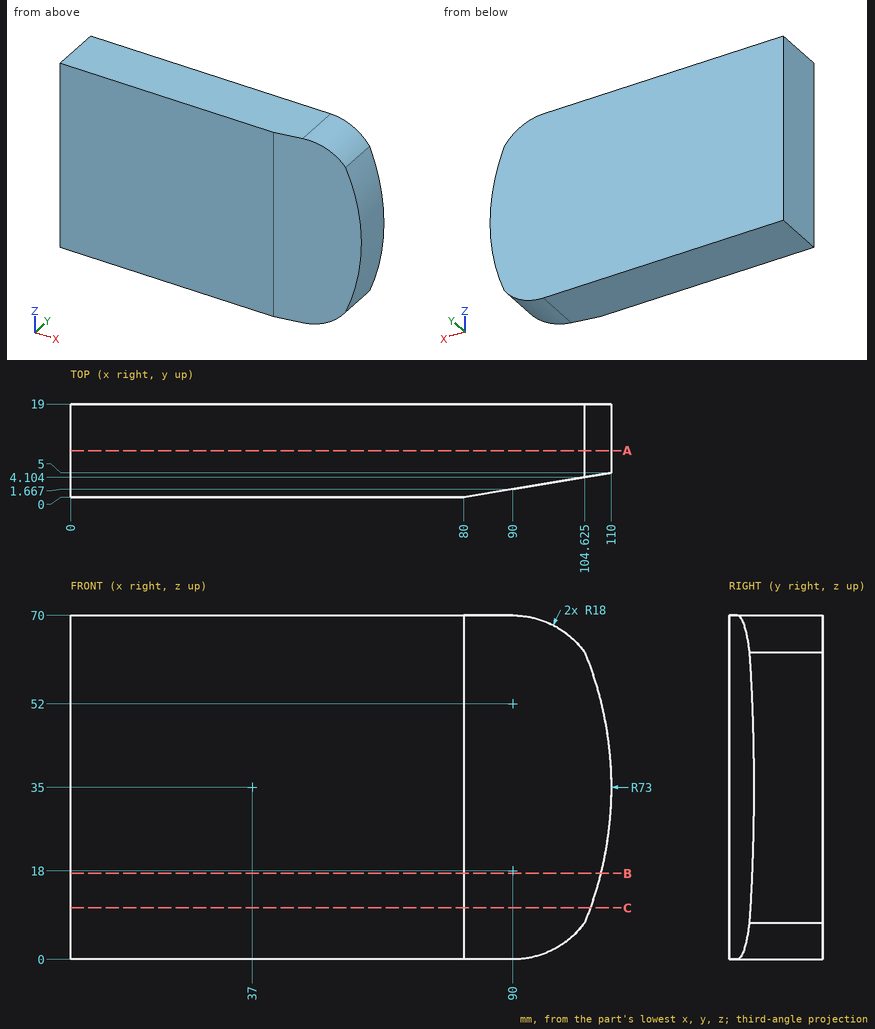
Design review of the part shown in the three views and the two pictorial views. Dimensions are in mm from the part's minimum x, y and z. Give positions to 0.01 mm unless a question says otherwise; leave off trailing zeros. Loops run counter-clockwise (first coordinate to the right, second up) from the corner with the lowest first, then second, coordinate; pieces in that order, holes last. Notation, with made-up numbers: (82.5, 37.25) -> (112.5, 37.25) arc R34 cw to (112.5, 70.25) -> close; hole circle Ø7 at (-6.5, 24.25). An arc over 180 degrees is marked (long way). Put each result on its own line as item: value. Start each with the question number.
1. We need section C-C on z = 10.5. State the section outline as (x, y) points (1 decimal), then the cut area to 3 significant figures.
2. We need section A-A on y = 9.5. State the section outline as (x, z) points (1 decimal), then the cut area to 3 significant figures.
3. Wall thickness on probe 1 along Y at (x, z) = (81.5, 38.5); probe 2 along X at (y, z) = (5, 56.5); probe 3 along X at (y, z) = (8, 31): over which ranges is each line inside the solid? List them lowest first.
4. We need section B-B on z = 17.5. State the section outline as (x, y) points (1 decimal).
5. Clearance check with a flat-ended pin moving along its axis: P1, Ø10, axis at y = 5.5, z = 7.5, coming from the -X side. State where the tip first meets the part, or that it passes through.
Determined:
1. outline: (0, 0) -> (80, 0) -> (105.8, 4.3) -> (105.8, 19) -> (0, 19) -> close
1. area: 1,950 mm^2
2. outline: (0, 0) -> (90, 0) arc R18 ccw to (104.6, 7.5) arc R73 ccw to (104.6, 62.5) arc R18 ccw to (90, 70) -> (0, 70) -> close
2. area: 7,460 mm^2
3. probe 1: 0.25 to 19
3. probe 2: 0 to 106.76
3. probe 3: 0 to 109.89
4. outline: (0, 0) -> (80, 0) -> (107.9, 4.6) -> (107.9, 19) -> (0, 19) -> close
5. P1: x = 0
